Can you work these out from the model? Positions are in its coordinate system, mm. Face numbers are marked on the shaded views. A direction names the side the tool comes from. Give positions to 0.01 mm unless a question says otherwise; leave off trailing zeros. Order: outer loops, then holes, each group sorted by start corner. A loop starts at its lowest first (then second) coordinate and runs counter-clockwise, first axis right, second up. Notation, with made-up numbers: (-40, 28) - (-36, 28) arc R27 cw to (-36, 67) - close; hole circle Ø9 at (69.5, 52.25). An arc over 180 degrees is marked (long way). Answer as a JSON object with one key per item and string values.
```python
from build123d import *

# Parameters (mm, degrees)
F0_R     = 20
F1_DEPTH = 13
F2_R     = 12.5
F3_DEPTH = 10
F4_R     = 3
F6_DEPTH = 7
F8_DEPTH = 25


with BuildPart() as f1:
    # F0 (on Top) → F1 (new body)
    with BuildSketch(Plane.XY):
        Circle(F0_R)
    extrude(amount=F1_DEPTH)

    # F2 (on face) → F3 (join)
    with BuildSketch(Plane.XY.offset(13)):
        Circle(F2_R)
    extrude(amount=F3_DEPTH)

    # F4
    f4_edges = [f1.edges().sort_by_distance(p)[0] for p in [
        (-20, 0, 13),
        (-20, 0, 0),
    ]]
    fillet(f4_edges, radius=F4_R)

    # F5 (on face) → F6 (cut)
    with BuildSketch(Plane.XY.offset(23)):
        Polygon((8.2705426061, 4.775), (0, 9.55), (-8.2705426061, 4.775), (-8.2705426061, -4.775), (0, -9.55), (8.2705426061, -4.775), align=None)
    extrude(amount=-F6_DEPTH, mode=Mode.SUBTRACT)

    # F7 (on face) → F8 (cut)
    with BuildSketch(Plane(origin=(0, 0, 0), x_dir=(1, 0, 0), z_dir=(0, 0, -1))):
        with BuildLine():
            ThreePointArc((14.7224318372, 8.5000000471), (16.435854573, 7.1334012872), (18.6214276605, 7.2967411826))
            ThreePointArc((18.6214276605, 7.2967411826), (17.3205080757, 10), (15.6298770592, 12.4782588174))
            ThreePointArc((15.6298770592, 12.4782588174), (14.3956340287, 10.6671670025), (14.7224318372, 8.5000000471))
        make_face()
        with BuildLine():
            ThreePointArc((20.3205080757, -10), (19.8604646456, -8.4035600159), (18.6214276605, -7.2967411826))
            ThreePointArc((18.6214276605, -7.2967411826), (17.3205080757, -10), (15.6298770592, -12.4782588174))
            ThreePointArc((15.6298770592, -12.4782588174), (18.7219549977, -12.6525358668), (20.3205080757, -10))
        make_face()
        with BuildLine():
            ThreePointArc((15.6298770592, -12.4782588174), (17.3205080757, -10), (18.6214276605, -7.2967411826))
            ThreePointArc((18.6214276605, -7.2967411826), (16.435854533, -7.1334012995), (14.7224317953, -8.5000001196))
            ThreePointArc((14.7224317953, -8.5000001196), (14.395634038, -10.6671670433), (15.6298770592, -12.4782588174))
        make_face()
        with BuildLine():
            ThreePointArc((-1.46e-08, 17), (2.040220571, 17.8005682502), (2.9915506013, 19.775))
            ThreePointArc((2.9915506013, 19.775), (0, 20), (-2.9915506013, 19.775))
            ThreePointArc((-2.9915506013, 19.775), (-2.0402205817, 17.8005682602), (-1.46e-08, 17))
        make_face()
        with BuildLine():
            ThreePointArc((-2.9915506013, 19.775), (0, 20), (2.9915506013, 19.775))
            ThreePointArc((2.9915506013, 19.775), (2.9978869061, 19.8874207031), (3, 20))
            ThreePointArc((3, 20), (-0.1125792969, 22.9978869061), (-2.9915506013, 19.775))
        make_face()
        with BuildLine():
            ThreePointArc((3, -20), (2.9978869061, -19.8874207031), (2.9915506013, -19.775))
            ThreePointArc((2.9915506013, -19.775), (0, -20), (-2.9915506013, -19.775))
            ThreePointArc((-2.9915506013, -19.775), (-0.1125792969, -22.9978869061), (3, -20))
        make_face()
        with BuildLine():
            ThreePointArc((-2.9915506013, -19.775), (0, -20), (2.9915506013, -19.775))
            ThreePointArc((2.9915506013, -19.775), (2.0402205635, -17.8005682433), (-3.5e-08, -17))
            ThreePointArc((-3.5e-08, -17), (-2.0402205891, -17.8005682671), (-2.9915506013, -19.775))
        make_face()
        with BuildLine():
            ThreePointArc((-18.6214276605, 7.2967411826), (-16.4358546167, 7.1334012737), (-14.7224318829, 8.4999999678))
            ThreePointArc((-14.7224318829, 8.4999999678), (-14.4227306016, 9.2235428467), (-14.3205080757, 10))
            ThreePointArc((-14.3205080757, 10), (-14.6679722089, 11.401446922), (-15.6298770592, 12.4782588174))
            ThreePointArc((-15.6298770592, 12.4782588174), (-17.3205080757, 10), (-18.6214276605, 7.2967411826))
        make_face()
        with BuildLine():
            ThreePointArc((-14.3205080757, -10), (-14.4227305909, -9.2235428867), (-14.7224318416, -8.5000000394))
            ThreePointArc((-14.7224318416, -8.5000000394), (-16.4358545772, -7.1334012859), (-18.6214276605, -7.2967411826))
            ThreePointArc((-18.6214276605, -7.2967411826), (-17.3205080757, -10), (-15.6298770592, -12.4782588174))
            ThreePointArc((-15.6298770592, -12.4782588174), (-14.6679722089, -11.401446922), (-14.3205080757, -10))
        make_face()
        with BuildLine():
            ThreePointArc((-18.6214276605, 7.2967411826), (-17.3205080757, 10), (-15.6298770592, 12.4782588174))
            ThreePointArc((-15.6298770592, 12.4782588174), (-19.918584287, 11.5), (-18.6214276605, 7.2967411826))
        make_face()
        with BuildLine():
            ThreePointArc((-18.6214276605, -7.2967411826), (-19.918584287, -11.5), (-15.6298770592, -12.4782588174))
            ThreePointArc((-15.6298770592, -12.4782588174), (-17.3205080757, -10), (-18.6214276605, -7.2967411826))
        make_face()
    extrude(amount=-F8_DEPTH, mode=Mode.SUBTRACT)


solid = f1.part
```
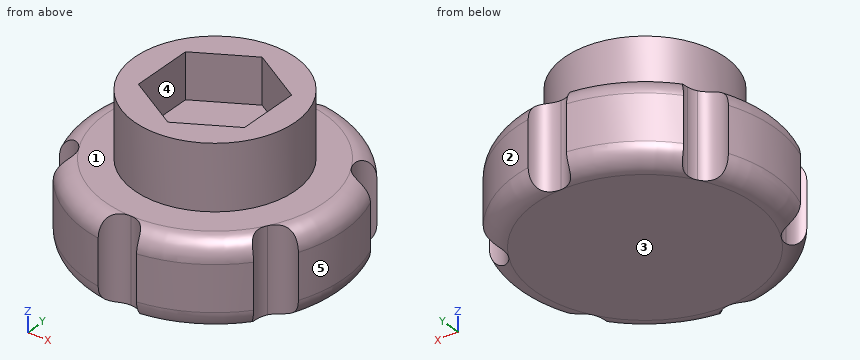
Q1. Which directions (+Z, -Z, +X, -X, +Y, -Y) give clear straight access to the entire face, cutting with the end or side of a thin tool? Please do the marked faces 1 and 2.
Recorded:
{"face 1": "+Z", "face 2": "+Z, -Z, +X, +Y"}
Q2. If we section it at B-B, the plane y = 0: Please give me the cut outline in (x, z).
Recorded:
{"outline": "(-20, 3) arc R3 ccw to (-17, 0) - (17, 0) arc R3 ccw to (20, 3) - (20, 10) arc R3 ccw to (17, 13) - (12.5, 13) - (12.5, 23) - (8.27, 23) - (8.27, 16) - (-8.27, 16) - (-8.27, 23) - (-12.5, 23) - (-12.5, 13) - (-17, 13) arc R3 ccw to (-20, 10) - close"}
Q3. I'm going to push flat-ended pins straight in: pin 1 Ø7.5 at (y, z) = (-0.5, 20) entering from +X; pin 2 Ø1.5 at (y, z) = (12.5, 3) entering from -X; pin 3 Ø2 at (y, z) = (-2.5, 18.5) entering from -X. Where does each tip first touch, or does it pass through?
Recorded:
{"pin 1": "stops at x = 12.5", "pin 2": "stops at x = -15.63", "pin 3": "stops at x = -12.41"}
Q4. If we section it at A-A, the plane z = 4.5: Please give me the cut outline in (x, y) (1 decimal), then the cut area to 3 significant figures.
Recorded:
{"outline": "(-18.6, -7.3) arc R3 cw to (-15.6, -12.5) arc R20 ccw to (-3, -19.8) arc R3 cw to (3, -19.8) arc R20 ccw to (15.6, -12.5) arc R3 cw to (18.6, -7.3) arc R20 ccw to (18.6, 7.3) arc R3 cw to (15.6, 12.5) arc R20 ccw to (3, 19.8) arc R3 cw to (-3, 19.8) arc R20 ccw to (-15.6, 12.5) arc R3 cw to (-18.6, 7.3) arc R20 ccw to start", "area": "1,170 mm^2"}
Q5. If we section it at C-C, the plane z = 12.25: Please give me the cut outline in (x, y).
Recorded:
{"outline": "(-17.64, -7.02) arc R3 cw to (-14.9, -11.77) arc R18.98 ccw to (-2.74, -18.79) arc R3 cw to (2.74, -18.79) arc R18.98 ccw to (14.9, -11.77) arc R3 cw to (17.64, -7.02) arc R18.98 ccw to (17.64, 7.02) arc R3 cw to (14.9, 11.77) arc R18.98 ccw to (2.74, 18.79) arc R3 cw to (-2.74, 18.79) arc R18.98 ccw to (-14.9, 11.77) arc R3 cw to (-17.64, 7.02) arc R18.98 ccw to start"}
Q6. I need wall thicknesses on L1, parallel to Z at x = -3.5, y = -16; L2, parallel to X at y = 0, z = 7; L3, parallel to Z at x = 3.5, y = -2.5. Which ranges of each line are inside material? Lowest first, please.
Recorded:
{"L1": "z = 0 to 13", "L2": "x = -20 to 20", "L3": "z = 0 to 16"}
Q7. We'd pull the mould along Y, two halves only. Please class the marked faces 3, 4 and 5: released by +Y, released by -Y, zero draft, split by the parting line, or undercut.
Recorded:
{"face 3": "zero draft", "face 4": "undercut", "face 5": "split by the parting line"}
